from build123d import *

# Parameters (mm, degrees)
SKETCH1_W           = 100
SKETCH1_H           = 100
SKETCH1_R           = 2.5
BOSS_EXTRUDE1_DEPTH = 6
FILLET1_R           = 3
FILLET2_R           = 3


with BuildPart() as part:
    # Sketch1 → Boss-Extrude1 (new body)
    with BuildSketch(Plane(origin=(0, 0, 0), x_dir=(1, 0, 0), z_dir=(0, 1, 0))):
        with Locations((40, 40)):
            Rectangle(SKETCH1_W, SKETCH1_H)
        Circle(SKETCH1_R, mode=Mode.SUBTRACT)
        with Locations((80, 0)):
            Circle(SKETCH1_R, mode=Mode.SUBTRACT)
        with Locations((0, 80)):
            Circle(SKETCH1_R, mode=Mode.SUBTRACT)
        with Locations((80, 80)):
            Circle(SKETCH1_R, mode=Mode.SUBTRACT)
        with Locations((22, 22)):
            Circle(SKETCH1_R, mode=Mode.SUBTRACT)
        with Locations((58, 22)):
            Circle(SKETCH1_R, mode=Mode.SUBTRACT)
        with Locations((22, 54)):
            Circle(SKETCH1_R, mode=Mode.SUBTRACT)
        with Locations((58, 54)):
            Circle(SKETCH1_R, mode=Mode.SUBTRACT)
    extrude(amount=BOSS_EXTRUDE1_DEPTH)

    # Fillet1
    fillet1_edges = [part.edges().sort_by_distance(p)[0] for p in [
        (90, 3, 10),
        (-10, 3, 10),
    ]]
    fillet(fillet1_edges, radius=FILLET1_R)

    # Fillet2
    fillet2_edges = [part.edges().sort_by_distance(p)[0] for p in [
        (-10, 3, -90),
        (90, 3, -90),
    ]]
    fillet(fillet2_edges, radius=FILLET2_R)


solid = part.part
Work out the finished part from the listing and answer in its coordinate system (mm). Round coordinates to 2 decimals unless told otherwise and drop trailing zeros. Loops run counter-clockwise (first coordinate to the right, second up) from the corner with the lowest first, then second, coordinate; pieces in that order, holes last. Notation, with made-up numbers: (49, -27.75) - (69, -27.75) arc R31 cw to (69, 9.25) - close; hole circle Ø11 at (-33.5, 42). An arc over 180 degrees is marked (long way). One line per item, written item: value.
Q1. Find section B-B on z = -80. Give the vertices of the cut face in (x, y), and give its area (3 significant figures).
Check values:
outline: (-10, 0) - (-2.5, 0) - (-2.5, 6) - (-10, 6) - close; (2.5, 0) - (77.5, 0) - (77.5, 6) - (2.5, 6) - close; (82.5, 0) - (90, 0) - (90, 6) - (82.5, 6) - close
area: 540 mm2
Q2. Find section C-C on y = 3.35. State how many separate pieces and enclosed holes the cut face has, and give its area (3 significant figures).
Check values:
separate pieces: 1
enclosed holes: 8
area: 9,840 mm2
Q3. Straight lines are drawn through the part: probe 1 along X at (y, z) = (1.6, -22); probe 2 along X at (y, z) = (2.05, -80); probe 3 along Z at (x, y) = (80, 2.35). For each, find the intervals that lie inside material, in ascending order.
Check values:
probe 1: -10 to 19.5, 24.5 to 55.5, 60.5 to 90
probe 2: -10 to -2.5, 2.5 to 77.5, 82.5 to 90
probe 3: -90 to -82.5, -77.5 to -2.5, 2.5 to 10
Q4. Find section A-A on x = 0. Give the vertices of the cut face in (y, z), and give its area (3 significant figures).
Check values:
outline: (0, -90) - (6, -90) - (6, -82.5) - (0, -82.5) - close; (0, -77.5) - (6, -77.5) - (6, -2.5) - (0, -2.5) - close; (0, 2.5) - (6, 2.5) - (6, 10) - (0, 10) - close
area: 540 mm2
Q5. The mould has two halves that part along X. Classify faces 1 (the flat face through (39, 6, -41)), 2 (the cylindrical face through (77.5, 3, -80.1)), 3 (the cylindrical face through (19.5, 3, -54.1)), 4 (the flat face through (-10, 3, -39)): +X half, -X half, draft (parallel to the pull), parting line (faces both ways), or undercut.
Check values:
face 1: draft
face 2: undercut
face 3: undercut
face 4: -X half
